Check sheet for the modelled part. Datum: model origin and axes. Units: mm. A direction names the side the tool comes from. Coordinates: 2 decimals unless noted, no trailing zeros. Loops run counter-clockwise (first coordinate to the right, second up) from the corner with the lowest first, then second, coordinate; pieces in that order, holes last. Notation, with made-up numbers: (-21, -12) - (21, -12) arc R15 cw to (21, 17) - close; hole circle Ø10 at (-15, -33.75). An arc over 180 degrees is marked (long way). Answer as a JSON object with one key per item and string values. Group by question number.
from build123d import *

# Parameters (mm, degrees)
SKETCH1_R           = 1.5
BOSS_EXTRUDE1_DEPTH = 3
SKETCH3_R           = 1.6
CUT_EXTRUDE1_DEPTH  = 3
SKETCH4_R           = 4
SKETCH4_R_2         = 1.6
BOSS_EXTRUDE2_DEPTH = 3
CUT_EXTRUDE2_DEPTH  = 3


with BuildPart() as part:
    # Sketch1 → Boss-Extrude1 (new body)
    with BuildSketch(Plane.XY):
        with BuildLine():
            Line((-26.877501001, -2.5), (30, -2.5))
            Line((30, -2.5), (30, 2.5))
            Line((30, 2.5), (-26.877501001, 2.5))
            ThreePointArc((-26.877501001, 2.5), (-34, 0), (-26.877501001, -2.5))
        make_face()
        with Locations((-30, 0)):
            Circle(SKETCH1_R, mode=Mode.SUBTRACT)
    extrude(amount=BOSS_EXTRUDE1_DEPTH)

    # Sketch3 → Cut-Extrude1 (cut)
    with BuildSketch(Plane.XY.offset(3)):
        with Locations((26.727711113, 0)):
            Circle(SKETCH3_R)
    extrude(amount=-CUT_EXTRUDE1_DEPTH, mode=Mode.SUBTRACT)

    # Sketch4 → Boss-Extrude2 (add)
    with BuildSketch(Plane.XY.offset(3)):
        with Locations((26.727711113, 0)):
            Circle(SKETCH4_R)
        with Locations((26.727711113, 0)):
            Circle(SKETCH4_R_2, mode=Mode.SUBTRACT)
    extrude(amount=-BOSS_EXTRUDE2_DEPTH)

    # Sketch5 → Cut-Extrude2 (cut)
    with BuildSketch(Plane.XY.offset(3)):
        with BuildLine():
            Line((30, 2.5), (29.850210112, 2.5))
            ThreePointArc((29.850210112, 2.5), (29.926661234, 2.4013992), (30, 2.300462005))
            Line((30, 2.300462005), (30, 2.5))
        make_face()
        with BuildLine():
            Line((30, -2.5), (30, -2.300462005))
            ThreePointArc((30, -2.300462005), (29.926661234, -2.4013992), (29.850210112, -2.5))
            Line((29.850210112, -2.5), (30, -2.5))
        make_face()
    extrude(amount=-CUT_EXTRUDE2_DEPTH, mode=Mode.SUBTRACT)


solid = part.part
1. Sectioned sample at B-B on y = 0. Record the cut outline in (x, z), plus the area to 3 significant figures.
2. Sectioned sample at A-A on x = -30. Record the cut outline in (y, z), plus the area to 3 significant figures.
3. Sectioned sample at C-C on z = 1.85. Record the cut outline in (x, y), plus the area to 3 significant figures.
4. Access from +Z, -Z, +X, -X, +Y, -Y to the whole of each face (thin tool, end or side, straight path). Record for faces 5 (the face through (-2, 0, 0)), 6 (the face through (-2, -2.5, 1)).
5. Gauge pin test, flat ends, axial feed: pin 1 (1.5 mm diameter, centred on x = 3, z = 1, fed in from +Y); pin 2 (3.5 mm diameter, centred on x = 26.73, y = 0, fed in from +Z); pin 3 (1.5 mm diameter, centred on x = 11, z = 2, fed in from -Y). Record the tip position at first contact, or that the pin passes through.
6. Sectioned sample at D-D on x = 7. Record the cut outline in (y, z).
7. Material ranges on line 1 (Y direction, x = -30, z = 1.2); line 2 (X direction, y = -0.75, z = 2.7); line 3 (X direction, y = 0.5, z = 1.9), recorded low to high.
8. Release check for a two-part mould opening along Y. For faces 1 (the face through (-1, 2.5, 1)), 2 (the face through (-31.5, 0.07, 1.48)), 3 (the face through (-2, 0, 3)), 4 (the face through (25.548, 1.081, 1.521)) record: released by +Y, released by -Y, zero draft, split by the parting line, or undercut.
Answers follow:
{
 "1": {"outline": "(-34, 0) - (-31.5, 0) - (-31.5, 3) - (-34, 3) - close; (-28.5, 0) - (25.13, 0) - (25.13, 3) - (-28.5, 3) - close; (28.33, 0) - (30.73, 0) - (30.73, 3) - (28.33, 3) - close", "area": "176 mm^2"},
 "2": {"outline": "(-4, 0) - (-1.5, 0) - (-1.5, 3) - (-4, 3) - close; (1.5, 0) - (4, 0) - (4, 3) - (1.5, 3) - close", "area": "15.0 mm^2"},
 "3": {"outline": "(-26.88, -2.5) - (23.61, -2.5) arc R4 ccw (long way) to (23.61, 2.5) - (-26.88, 2.5) arc R4 ccw (long way) to start; hole circle Ø3 at (-30, 0); hole circle Ø3.2 at (26.73, 0)", "area": "332 mm^2"},
 "4": {"face 5": "-Z, +X, -X, +Y, -Y", "face 6": "+Z, -Z, -Y"},
 "5": {"pin 1": "stops at y = 2.5", "pin 2": "stops at z = 3", "pin 3": "stops at y = -2.5"},
 "6": {"outline": "(-2.5, 0) - (2.5, 0) - (2.5, 3) - (-2.5, 3) - close"},
 "7": {"line 1": "y = -4 to -1.5, 1.5 to 4", "line 2": "x = -33.93 to -31.3, -28.7 to 25.31, 28.14 to 30.66", "line 3": "x = -33.97 to -31.41, -28.59 to 25.21, 28.25 to 30.7"},
 "8": {"face 1": "released by +Y", "face 2": "undercut", "face 3": "zero draft", "face 4": "undercut"}
}
